```python
from build123d import *

# Parameters (mm, degrees)
SALIENTE_EXTRUIR1_DEPTH = 10
CROQUIS2_R              = 1.5
SALIENTE_EXTRUIR2_DEPTH = 6.7
CROQUIS3_R              = 1.5
CORTAR_EXTRUIR1_DEPTH   = 7


with BuildPart() as part:
    # Croquis1 → Saliente-Extruir1 (new body)
    with BuildSketch(Plane.XY):
        Polygon((2.655811238, 0), (1.327905619, 2.3), (-1.327905619, 2.3), (-2.655811238, 0), (-1.327905619, -2.3), (1.327905619, -2.3), align=None)
    extrude(amount=SALIENTE_EXTRUIR1_DEPTH)

    # Croquis2 → Saliente-Extruir2 (add)
    with BuildSketch(Plane(origin=(0, 0, 0), x_dir=(-1, 0, 0), z_dir=(0, 0, -1))):
        Circle(CROQUIS2_R)
    extrude(amount=SALIENTE_EXTRUIR2_DEPTH)

    # Croquis3 → Cortar-Extruir1 (cut)
    with BuildSketch(Plane.XY.offset(10)):
        Circle(CROQUIS3_R)
    extrude(amount=-CORTAR_EXTRUIR1_DEPTH, mode=Mode.SUBTRACT)


solid = part.part
```
Could you check a few things on this model? Use its own coordinates, in mm. A direction names the side the tool comes from. Coordinates: 2 decimals unless noted, no trailing zeros. Write each loop counter-clockwise with the first axis right and the second up, starting at its lowest first coordinate (ties: lowest second). Pieces come first, ordered by that corner, then holes. Notation, with made-up numbers: (-19, 88.5) - (4, 88.5) arc R26 cw to (4, 115.5) - close; hole circle Ø6 at (-21.75, 46.5). An arc over 180 degrees is marked (long way). Use a Markdown table: item, result.
Q1. Please list where these lines run through material, in increasing order: L1, parallel to Y at x = 0, z = 8.25; L2, parallel to Z at x = 2.4, y = 0.25; L3, parallel to Z at x = -0.35, y = 0.2.
Geometry check:
| item | result |
|---|---|
| L1 | y = -2.3 to -1.5, 1.5 to 2.3 |
| L2 | z = 0 to 10 |
| L3 | z = -6.7 to 3 |
Q2. Imagine slicing it at A-A (z = 8). List the corners of the cut face in (x, y) for me.
Geometry check:
| item | result |
|---|---|
| outline | (-2.66, 0) - (-1.33, -2.3) - (1.33, -2.3) - (2.66, 0) - (1.33, 2.3) - (-1.33, 2.3) - close; hole circle Ø3 at (0, 0) |
Q3. I'm going to push a flat-ended pin straight in: pin 1 Ø3 at (x, z) = (1, -1) entering from -Y. Where does the tip first touch, or does it pass through?
Geometry check:
| item | result |
|---|---|
| pin 1 | stops at y = -2.3 |
Q4. Imagine slicing it at C-C (y = 0.35). List the corners of the cut face in (x, z) for me, and give its area (3 significant figures).
Geometry check:
| item | result |
|---|---|
| outline | (-2.45, 0) - (-1.46, 0) - (-1.46, -6.7) - (1.46, -6.7) - (1.46, 0) - (2.45, 0) - (2.45, 10) - (1.46, 10) - (1.46, 3) - (-1.46, 3) - (-1.46, 10) - (-2.45, 10) - close |
| area | 48.2 mm2 |
Q5. Which directions (+Z, -Z, +X, -X, +Y, -Y) give clear straight access to the entire face, cutting with the end or side of a thin tool? Please do faces 4 (the flat face through (0, 2, 0)), 5 (the cylindrical face through (-1.5, 0.07, 6.55)), 6 (the flat face through (0, 0, -6.7)).
Geometry check:
| item | result |
|---|---|
| face 4 | -Z |
| face 5 | +Z |
| face 6 | -Z, +X, -X, +Y, -Y |
Q6. Thinking about a two-plate mould opening in Y: for faces 1 (the flat face through (0, 0, 3)), 2 (the flat face through (0, 2.3, 5)), 3 (the cylindrical face through (1.5, 0.07, -3.3)), which applies, +Y half, -Y half, draft (parallel to the pull), parting line (faces both ways), or undercut?
Geometry check:
| item | result |
|---|---|
| face 1 | undercut |
| face 2 | +Y half |
| face 3 | parting line |
Q7. Imagine slicing it at B-B (x = 0). List the corners of the cut face in (y, z) for me.
Geometry check:
| item | result |
|---|---|
| outline | (-2.3, 0) - (-1.5, 0) - (-1.5, -6.7) - (1.5, -6.7) - (1.5, 0) - (2.3, 0) - (2.3, 10) - (1.5, 10) - (1.5, 3) - (-1.5, 3) - (-1.5, 10) - (-2.3, 10) - close |
Q8. Imagine slicing it at D-D (z = -5.5). List the corners of the cut face in (x, y) for me.
Geometry check:
| item | result |
|---|---|
| outline | circle Ø3 at (0, 0) |
